Verification items for this drawing (mm, ordinates from the low corner). A direction names the side the tool comes from. Round coordinates to 2 decimals unless told otherwise and drop trailing zeros. Order: outer loops, then holes, each group sorted by start corner. A loop starts at its lowest first (then second) coordinate and runs counter-clockwise, first axis right, second up. Notation, with made-up numbers: (-19.5, -28) -> (10.5, -28) arc R15 cw to (10.5, -4) -> close; hole circle Ø1 at (-27.5, 12.25). An arc over 180 degrees is marked (long way). Answer in a Markdown table with one row per item. Add a question column.
1. Sectioned sample at D-D, the plane z = 16. Record the boundary of the cut face in (x, y), then the cut area to 3 significant figures.
2. Draft check along X on the marked faces 1, 2, 3 and 4. Enter one of: +X half, -X half, draft (parallel to the pull), parting line (faces both ways), or undercut.
3. Sectioned sample at C-C, the plane z = 5.25. Record the boundary of the cut face in (x, y).
4. Depth check by flat-ended pin: P1, Ø6, axis at x = 5.5, z = 16.5, coming from the -Y side; P2, Ø8, axis at y = 18, z = 21.5, coming from the +X side; P3, Ø1.5, axis at y = 3.5, z = 25.5, coming from the -X side. Enter the tip coordinate at first touch or a pass-through.
5. Material ranges on L1, parallel to Z at x = 15, y = 23.25; L2, parallel to X at y = 5.5, z = 26.25 (1 decimal); L3, parallel to Z at x = 22.25, y = 14.5 (1 decimal), recorded low to high. Write a range as from..to.
6. Access from +Z, -Z, +X, -X, +Y, -Y to the whole of each face (thin tool, end or side, straight path). Record for the marked faces 5, 6 and 7.
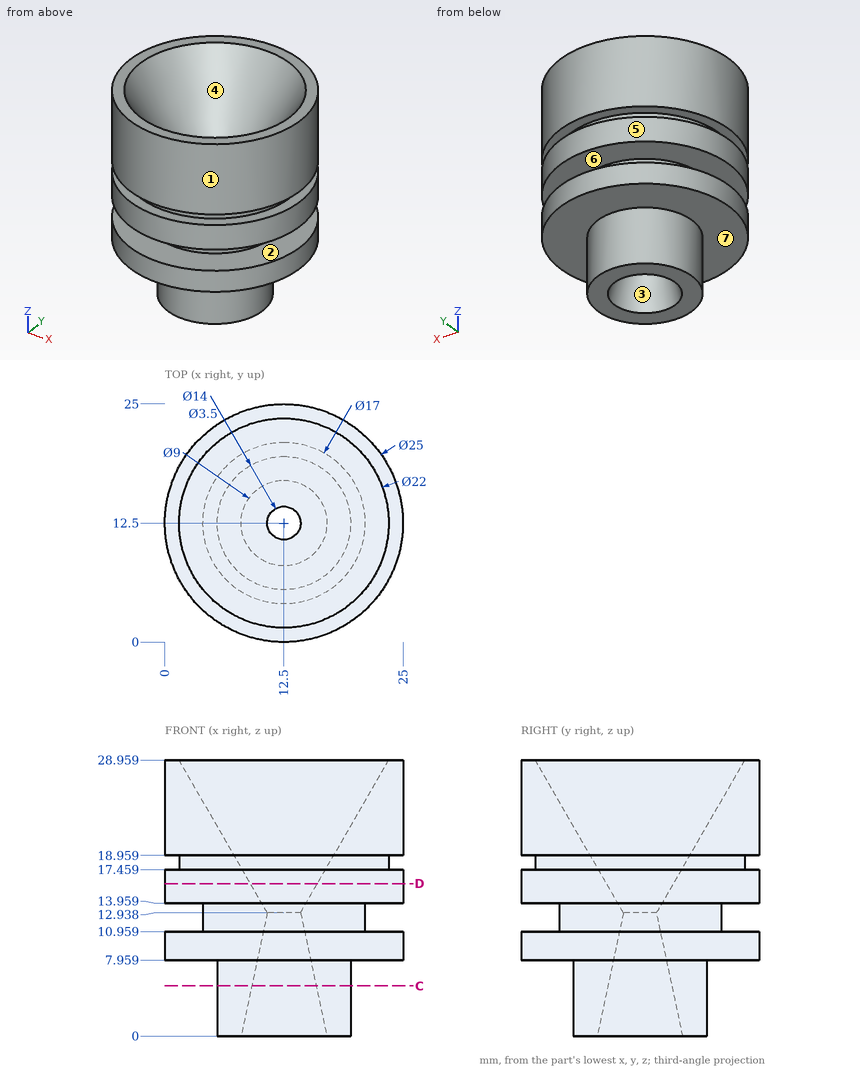
Answer key:
| question | item | result |
|---|---|---|
| 1 | outline | circle Ø25 at (12.5, 12.5); hole circle Ø7.04 at (12.5, 12.5) |
| 1 | area | 452 mm² |
| 2 | face 1 | parting line |
| 2 | face 2 | draft |
| 2 | face 3 | undercut |
| 2 | face 4 | undercut |
| 3 | outline | circle Ø14 at (12.5, 12.5); hole circle Ø6.77 at (12.5, 12.5) |
| 4 | P1 | stops at y = 0.66 |
| 4 | P2 | stops at x = 24.91 |
| 4 | P3 | stops at x = 3.11 |
| 5 | L1 | z = 7.96..10.96, 13.96..17.46, 18.96..28.96 |
| 5 | L2 | x = 2.1..6.2, 18.8..22.9 |
| 5 | L3 | z = 8..11, 14..27.1 |
| 6 | face 5 | +Z, -Z |
| 6 | face 6 | none |
| 6 | face 7 | -Z |
